Check sheet for the modelled part. Datum: model origin and axes. Units: mm. A direction names the side the tool comes from. Give positions to 0.01 mm unless a question says otherwise; leave off trailing zeros. Order: outer loops, then holes, each group sorted by start corner. A loop starts at its lowest first (then second) coordinate and runs counter-clockwise, first axis right, second up. Notation, with made-up numbers: (31.25, -7.5) - (77.25, -7.5) arc R27 cw to (77.25, 15.5) - close; hole circle Ø1 at (-22, -28.5). An arc over 180 degrees is marked (long way). Answer in a Markdown table with one row per item.
Autodesk Inventor part; units mm, degrees
ref_plane "YZ Plane" through (0, 0, 0) normal (1, 0, 0) x (0, 1, 0)
ref_plane "XZ Plane" through (0, 0, 0) normal (0, 1, 0) x (-1, 0, 0)
ref_plane "XY Plane" through (0, 0, 0) normal (0, 0, 1) x (1, 0, 0)
sketch "Skizze1" plane through (0, 0, 0) normal (0, 0, 1) x (1, 0, 0)
  line L0 (-8, 10.5) -> (8, 10.5)
  line L1 (8, 10.5) -> (8, -10.5)
  line L2 (8, -10.5) -> (-8, -10.5)
  line L3 (-8, -10.5) -> (-8, 10.5)
  line L4 (0, 14.7) -> (0, -14.7)
  line L5 (-11.2, 0) -> (11.2, 0)
  point P0 (0, 0)
  dimension "d0" = 16
  dimension "d2" = 21
extrude "Extrusion1" add sketch "Skizze1" along normal blind 14
sketch "Skizze2" plane through (-8, -10.5, 0) normal (0, -1, 0) x (1, 0, 0)
  line L0 (2, 11) -> (14, 11)
  line L1 (14, 11) -> (14, 3.8)
  line L2 (2, 3.8) -> (2, 11)
  line L3 (10.5, 3.8) -> (10.5, 0.8)
  line L4 (10.5, 0.8) -> (5.5, 0.8)
  line L5 (5.5, 0.8) -> (5.5, 3.8)
  line L6 (16, 0) -> (0, 0)
  line L7 (16, 0) -> (16, 14)
  line L8 (0, 14) -> (16, 14)
  line L9 (0, 0) -> (0, 14)
  line L10 (8, 14) -> (8, 0) construction
  line L11 (14, 3.8) -> (10.5, 3.8)
  line L12 (5.5, 3.8) -> (2, 3.8)
  dimension "d5" = 3
  dimension "d6" = 0.8
  dimension "d8" = 2
  dimension "d9" = 5
  dimension "d10" = 3
extrude "Extrusion2" cut sketch "Skizze2" against normal blind 10 contours L0 L1 L11 L3 L4 L5 L12 L2
sketch "Skizze3" plane through (0, 0, 0) normal (0, 0, -1) x (-1, 0, 0)
  line L0 (-8, -10.5) -> (8, -10.5)
  line L1 (-8, 10.5) -> (-8, -10.5)
  line L2 (8, -10.5) -> (8, 10.5)
  line L3 (-5.7, 0) -> (5.7, 0) construction
  line L4 (0, -14.7) -> (0, 14.7) construction
  circle A0 centre (-5.7, 0) radius 1.5
  circle A1 centre (5.7, 0) radius 1.5
  point P0 (0, 0)
  dimension "d13" = 10.5
  dimension "d14" = 11.4
  dimension "d15" = 3
  dimension "d16" = 3
extrude "Extrusion3" add sketch "Skizze3" along normal blind 3.2 draft -5
sketch "Skizze4" plane through (-8, -10.5, 0) normal (-1, 0, 0) x (0, 0, 1)
  line L0 (14, 21) -> (14, 0)
  arc A0 (14, 0) -> (14, 8) centre (6.5, 4) ccw
  line L1 (14, 0) -> (14, 8)
  point P0 (0, 10.5)
  dimension "d19" = 1
  dimension "d20" = 8
extrude "Extrusion4" add sketch "Skizze4" against normal blind 16
sketch "Skizze5" plane through (0, 0, 14) normal (0, 0, 1) x (1, 0, 0)
  line L0 (-8, 10.5) -> (-8, -10.5)
  line L1 (8, -10.5) -> (8, 10.5)
  arc A0 (-8, -2.5) -> (-8, -10.5) centre (-0.5, -6.5) ccw
  line L2 (-8, -10.5) -> (-8, -2.5)
  point P0 (0, 0)
  dimension "d23" = 1
  dimension "d24" = 8
extrude "Extrusion5" add sketch "Skizze5" against normal blind 14
mirror "Spiegeln1" about plane through (0, 0, 0) normal (1, 0, 0) of "Extrusion5"
properties part number "RJ45 Socket" material "Aluminium 6061"
(1) Cross-section at D-D, the plane y = -9. Record the cut outline in (x, z).
Geometry says:
| item | result |
|---|---|
| outline | (-8.62, 0) - (8.62, 0) - (8.62, 14) - (8, 14) - (8, 14.62) - (-8, 14.62) - (-8, 14) - (-8.62, 14) - close; hole (-6, 3.8) - (-2.5, 3.8) - (-2.5, 0.8) - (2.5, 0.8) - (2.5, 3.8) - (6, 3.8) - (6, 11) - (-6, 11) - close |
(2) Access from +Z, -Z, +X, -X, +Y, -Y to the whole of each face (thin tool, end or side, straight path). Record for faces 4 (the flat face through (4, -6, 3.8)), 5 (the flat face through (-8.4, -6.4, 14)), 6 (the flat face through (8, -6.4, 14.4)).
Geometry says:
| item | result |
|---|---|
| face 4 | -Y |
| face 5 | +Z, -X, +Y, -Y |
| face 6 | +Z, +X, +Y, -Y |
(3) Cross-section at B-B, the plane z = 9. Record the cut outline in (x, y), then the cut area to 3 significant figures.
Geometry says:
| item | result |
|---|---|
| outline | (-8, -10.5) - (-6, -10.5) - (-6, -0.5) - (6, -0.5) - (6, -10.5) - (8, -10.5) arc R8.5 ccw to (8, -2.5) - (8, 10.5) - (-8, 10.5) - (-8, -2.5) arc R8.5 ccw to start |
| area | 227 mm² |
(4) Cross-section at A-A, the plane x = -5.7. Record the cut outline in (y, z), then the cut area to 3 significant figures.
Geometry says:
| item | result |
|---|---|
| outline | (-10.5, 0) - (-1.5, 0) - (-1.22, -3.2) - (1.22, -3.2) - (1.5, 0) - (10.5, 0) - (10.5, 14) - (-2.5, 14) arc R8.5 ccw to (-10.5, 14) - (-10.5, 11) - (-0.5, 11) - (-0.5, 3.8) - (-10.5, 3.8) - close |
| area | 236 mm² |
(5) Thickness scan on L1, parallel to X at y = -1, z = 2.5; L2, parallel to Z at x = 0, y = -1; L3, parallel to Z at x = -3, y = -6.75. Record the ranges inside material, lowest first.
Geometry says:
| item | result |
|---|---|
| L1 | -8 to -2.5, 2.5 to 8 |
| L2 | 0 to 0.8, 11 to 14 |
| L3 | 0 to 3.8, 11 to 15 |
(6) Gauge pin test, flat ends, axial feed: P1, Ø1, axis at x = 3.5, y = -4, coming from the +Z side; P2, Ø4, axis at y = 2, z = 7, coming from the -X side; P3, Ø1.1, axis at y = -7.5, z = 14.5, coming from the -X side (3 decimals). Record the tip position at first contact, or that the pin passes through.
Geometry says:
| item | result |
|---|---|
| P1 | z = 14.76 |
| P2 | x = -8 |
| P3 | x = -8.965 |
(7) Cross-section at C-C, the plane y = 0. Record the cut outline in (x, z), then the cut area to 3 significant figures.
Geometry says:
| item | result |
|---|---|
| outline | (-8, 0) - (-7.2, 0) - (-6.92, -3.2) - (-4.48, -3.2) - (-4.2, 0) - (4.2, 0) - (4.48, -3.2) - (6.92, -3.2) - (7.2, 0) - (8, 0) - (8, 14) - (-8, 14) - close |
| area | 241 mm² |
(8) Mould release check, pull along Z, two halves, no side actions. Record for faces 1 (the flat face through (-6, 0, -3.2)), 2 (the flat face through (0, -0.5, 7)), 3 (the cylindrical face through (-0.1, -6.6, 15)): pulls with the +Z half, pulls with the -Z half, needs draft (parallel to the pull), parting line crosses it, or undercut.
Geometry says:
| item | result |
|---|---|
| face 1 | pulls with the -Z half |
| face 2 | undercut |
| face 3 | pulls with the +Z half |
